Read the model definition and answer for the solid it produces. Units are mm, in the model's axes. A direction names the side the tool comes from. Give positions to 0.01 mm unless a question says otherwise; leave off trailing zeros. Loops run counter-clockwise (first coordinate to the right, second up) from the corner with the lowest first, then second, coordinate; pieces in that order, holes last.
(1) Find section A-A, the plane z = -3. Write down the section's boundary in (x, y), then the cut area to 3 significant figures.
(2) Which of the six approach directions +Z, -Z, +X, -X, +Y, -Y give full straight-line access (tool end or side, diameter ignored) to faces 5 (the face through (8.355, 10.806, -35.969)), 6 (the face through (40, 4, -56)), 7 (the face through (32.25, 2, -27)), 8 (the face through (40.2, -3.5, -31.4)), 9 (the face through (69, 3, 0))?
(3) Find section D-D, the plane z = -14. Write down the section's boundary in (x, y), then the cut area to 3 significant figures.
(4) Straight lines are drawn through the part: probe 1 along Z at (x, y) = (45.5, 4); probe 2 along X at (y, z) = (4.5, -36.5); probe 3 along Z at (x, y) = (63, 6.5). For each, find the intervals that lie inside material, in ascending order.
(5) Find section B-B, the plane x = 40. Write down the section's boundary in (y, z), then the cut area to 3 significant figures.
(6) Determine the mould class of faces 1 (the face through (78.947, 10.806, -22.671)), 2 (the face through (40, -3, -61.906)), 3 (the face through (-7.454, 3.796, -33.947)), 4 (the face through (22.52, 4.19, -42.54)) for opening direction X: pulls with the +X half, pulls with the -X half, needs draft (parallel to the pull), parting line crosses it, or undercut.
(7) Find section C-C, the plane y = -2.5. Write down the section's boundary in (x, z).
(8) Each of these flat-tipped pins is pushed along its axis until it touches: P1, Ø1.5, axis at x = 73, z = -39.5, coming from the -Y side; P2, Ø4, axis at x = 32.5, z = -20.5, coming from the +Y side; P3, Ø3, axis at y = 9.5, z = -38.5, coming from the -X side; P4, Ø3, axis at x = 11.5, y = 4.5, coming from the +Z side. Where does it stop, or does it pass through?
```python
from build123d import *

# Parameters (mm, degrees)
EXTRUDE_1_DEPTH      = 14
CUT_EXTRUDE_START    = -6.3
CUT_EXTRUDE_1_DEPTH  = 6.3
CUT_EXTRUDE_START_2  = -3
CUT_EXTRUDE_2_DEPTH  = 3
SKETCH_4_R           = 6.01
CUT_EXTRUDE_3_DEPTH  = 2.9
CUT_EXTRUDE_4_REACH  = 109.588
SKETCH_5_R           = 2.6
CUT_EXTRUDE_START_3  = -1
SKETCH_6_R           = 4.6
CUT_EXTRUDE_6_DEPTH  = 1
EXTRUDE_2_DEPTH      = 5
SKETCH_8_R           = 11.5
CUT_EXTRUDE_7_DEPTH  = 4
CUT_EXTRUDE_8_REACH  = 110.373
SKETCH_9_R           = 1.8
FILLET_1_R           = 3
SKETCH_12_R          = 10
CUT_EXTRUDE_10_DEPTH = 8
EXTRUDE_3_DEPTH      = 61.90646084
SKETCH_19_R          = 6
CUT_EXTRUDE_14_DEPTH = 9
CUT_EXTRUDE_11_REACH = 108.687
SKETCH_13_R          = 5
SKETCH_21_R          = 15
CUT_EXTRUDE_15_DEPTH = 3
SKETCH_23_R          = 1.5
CUT_EXTRUDE_16_DEPTH = 7
CUT_EXTRUDE_START_4  = -5
CUT_EXTRUDE_19_DEPTH = 5
SKETCH_34_W          = 15.5
SKETCH_34_H          = 47.251878887
CUT_EXTRUDE_20_DEPTH = 3


with BuildPart() as part:
    # 草图1 → 凸台-拉伸1 (new body)
    with BuildSketch(Plane(origin=(0, 0, 0), x_dir=(1, 0, 0), z_dir=(0, 1, 0))):
        with BuildLine():
            Line((13.709398988, 61.90646084), (-5.160444431, 39.418257154))
            ThreePointArc((-5.160444431, 39.418257154), (-7.461946981, 33.861938484), (-6.160254038, 27.990381057))
            Line((-6.160254038, 27.990381057), (10, 0))
            Line((10, 0), (70, 0))
            Line((70, 0), (86.160254038, 27.990381057))
            ThreePointArc((86.160254038, 27.990381057), (87.414448614, 34.295642979), (84.571067812, 40.061448869))
            Line((84.571067812, 40.061448869), (66.290601012, 61.90646084))
            Line((66.290601012, 61.90646084), (13.709398988, 61.90646084))
        make_face()
    extrude(amount=EXTRUDE_1_DEPTH)

    # 草图2 → 切除-拉伸1 (cut)
    with BuildSketch(Plane(origin=(0, 14, 0), x_dir=(1, 0, 0), z_dir=(0, 1, 0)).offset(CUT_EXTRUDE_START)):
        with BuildLine():
            Line((-3.314954576, 23.062177826), (1.303847577, 23.062177826))
            Line((1.303847577, 23.062177826), (12.309401077, 4))
            Line((12.309401077, 4), (67.690598923, 4))
            Line((67.690598923, 4), (78.696152423, 23.062177826))
            Line((78.696152423, 23.062177826), (83.314954576, 23.062177826))
            Line((83.314954576, 23.062177826), (86.160254038, 27.990381057))
            ThreePointArc((86.160254038, 27.990381057), (87.461946981, 33.861938484), (85.160444431, 39.418257154))
            ThreePointArc((85.160444431, 39.418257154), (84.872773368, 39.746283133), (84.571067812, 40.061448869))
            Line((84.571067812, 40.061448869), (73.343672408, 53.478096796))
            Line((73.343672408, 53.478096796), (72.5, 54.486278592))
            Line((72.5, 54.486278592), (72.5, 35.067052168))
            Line((72.5, 35.067052168), (67.5, 35.067052168))
            Line((67.5, 35.067052168), (67.5, 46.251878887))
            Line((67.5, 46.251878887), (12.5, 46.251878887))
            Line((12.5, 46.251878887), (12.5, 35.067052168))
            Line((12.5, 35.067052168), (7.5, 35.067052168))
            Line((7.5, 35.067052168), (7.5, 54.506387288))
            Line((7.5, 54.506387288), (-5.160444431, 39.418257154))
            ThreePointArc((-5.160444431, 39.418257154), (-7.461946981, 33.861938484), (-6.160254038, 27.990381057))
            Line((-6.160254038, 27.990381057), (-3.314954576, 23.062177826))
        make_face()
    extrude(amount=CUT_EXTRUDE_1_DEPTH, mode=Mode.SUBTRACT)

    # 草图3 → 切除-拉伸2 (cut)
    with BuildSketch(Plane(origin=(0, 7.7, 0), x_dir=(1, 0, 0), z_dir=(0, 1, 0)).offset(CUT_EXTRUDE_START_2)):
        with BuildLine():
            Line((67.690598923, 4), (78.696152423, 23.062177826))
            ThreePointArc((78.696152423, 23.062177826), (70.865300468, 25.508351779), (67.5, 32.990381057))
            Line((67.5, 32.990381057), (67.5, 35.067052168))
            Line((67.5, 35.067052168), (67.5, 46.251878887))
            Line((67.5, 46.251878887), (12.5, 46.251878887))
            Line((12.5, 46.251878887), (12.5, 35.067052168))
            Line((12.5, 35.067052168), (12.5, 32.990381057))
            ThreePointArc((12.5, 32.990381057), (9.134699532, 25.508351779), (1.303847577, 23.062177826))
            Line((1.303847577, 23.062177826), (12.309401077, 4))
            Line((12.309401077, 4), (67.690598923, 4))
        make_face()
    extrude(amount=CUT_EXTRUDE_2_DEPTH, mode=Mode.SUBTRACT)

    # 草图4 → 切除-拉伸3 (cut)
    with BuildSketch(Plane(origin=(0, 7.7, 0), x_dir=(1, 0, 0), z_dir=(0, 1, 0))):
        with Locations(Location((2.5, 32.990381057, 0), (0, 0, 270))):
            Circle(SKETCH_4_R)
        with Locations(Location((77.5, 32.990381057, 0), (0, 0, 270))):
            Circle(SKETCH_4_R)
    extrude(amount=-CUT_EXTRUDE_3_DEPTH, mode=Mode.SUBTRACT)

    # 草图5 → 切除-拉伸4 (cut, up to next)
    with BuildSketch(Plane(origin=(0, 4.7, 0), x_dir=(1, 0, 0), z_dir=(0, 1, 0)), mode=Mode.PRIVATE) as cut_extrude_4_sk1:
        with Locations(Location((19.414467174, 39.146743637, 0), (0, 0, 270))):
            Circle(SKETCH_5_R)
    cut_extrude_4_tool1 = extrude(cut_extrude_4_sk1.sketch, amount=-CUT_EXTRUDE_4_REACH, mode=Mode.PRIVATE) & part.part
    # 草图5 → 切除-拉伸4 (cut, up to next)
    with BuildSketch(Plane(origin=(0, 4.7, 0), x_dir=(1, 0, 0), z_dir=(0, 1, 0)), mode=Mode.PRIVATE) as cut_extrude_4_sk2:
        with Locations(Location((60.585532826, 39.146743637, 0), (0, 0, 270))):
            Circle(SKETCH_5_R)
    cut_extrude_4_tool2 = extrude(cut_extrude_4_sk2.sketch, amount=-CUT_EXTRUDE_4_REACH, mode=Mode.PRIVATE) & part.part
    add(cut_extrude_4_tool1.solids().sort_by_distance((19.414467, 4.7, -39.146744))[0], mode=Mode.SUBTRACT)
    add(cut_extrude_4_tool2.solids().sort_by_distance((60.585533, 4.7, -39.146744))[0], mode=Mode.SUBTRACT)

    # 草图6 → 切除-拉伸6 (cut)
    with BuildSketch(Plane(origin=(0, 4.7, 0), x_dir=(1, 0, 0), z_dir=(0, 1, 0)).offset(CUT_EXTRUDE_START_3)):
        with BuildLine():
            Line((67.690598923, 4), (78.696152423, 23.062177826))
            ThreePointArc((78.696152423, 23.062177826), (70.865300468, 25.508351779), (67.5, 32.990381057))
            Line((67.5, 32.990381057), (67.5, 46.251878887))
            Line((67.5, 46.251878887), (12.5, 46.251878887))
            Line((12.5, 46.251878887), (12.5, 32.990381057))
            ThreePointArc((12.5, 32.990381057), (9.134699532, 25.508351779), (1.303847577, 23.062177826))
            Line((1.303847577, 23.062177826), (12.309401077, 4))
            Line((12.309401077, 4), (67.690598923, 4))
        make_face()
        with Locations(Location((19.414467174, 39.146743637, 0), (0, 0, 270))):
            Circle(SKETCH_6_R, mode=Mode.SUBTRACT)
        with Locations(Location((60.585532826, 39.146743637, 0), (0, 0, 270))):
            Circle(SKETCH_6_R, mode=Mode.SUBTRACT)
    extrude(amount=CUT_EXTRUDE_6_DEPTH, mode=Mode.SUBTRACT)

    # 草图7 → 凸台-拉伸2 (add)
    with BuildSketch(Plane.XY):
        with BuildLine():
            Line((10, 14), (70, 14))
            ThreePointArc((70, 14), (40, -16), (10, 14))
        make_face()
    extrude(amount=EXTRUDE_2_DEPTH)

    # 草图8 → 切除-拉伸7 (cut)
    with BuildSketch(Plane.XY.offset(5)):
        with Locations((40, 14)):
            Circle(SKETCH_8_R)
    extrude(amount=-CUT_EXTRUDE_7_DEPTH, mode=Mode.SUBTRACT)

    # 草图9 → 切除-拉伸8 (cut, up to next)
    with BuildSketch(Plane(origin=(0, 0, 0), x_dir=(-1, 0, 0), z_dir=(0, 0, -1)), mode=Mode.PRIVATE) as cut_extrude_8_sk1:
        with Locations((-55, -6)):
            Circle(SKETCH_9_R)
    cut_extrude_8_tool1 = extrude(cut_extrude_8_sk1.sketch, amount=-CUT_EXTRUDE_8_REACH, mode=Mode.PRIVATE) & part.part
    # 草图9 → 切除-拉伸8 (cut, up to next)
    with BuildSketch(Plane(origin=(0, 0, 0), x_dir=(-1, 0, 0), z_dir=(0, 0, -1)), mode=Mode.PRIVATE) as cut_extrude_8_sk2:
        with Locations((-25, -6)):
            Circle(SKETCH_9_R)
    cut_extrude_8_tool2 = extrude(cut_extrude_8_sk2.sketch, amount=-CUT_EXTRUDE_8_REACH, mode=Mode.PRIVATE) & part.part
    add(cut_extrude_8_tool1.solids().sort_by_distance((55, -6, 0))[0], mode=Mode.SUBTRACT)
    add(cut_extrude_8_tool2.solids().sort_by_distance((25, -6, 0))[0], mode=Mode.SUBTRACT)

    # 圆角1
    # the kernel refuses this fillet: 3 mm, written as the material it takes off along each edge
    with BuildSketch(Plane(origin=(78.696152423, 7.7, -23.062177826), x_dir=(1, 0, 0), z_dir=(0, 1, 0))) as fillet_1_piece_1:
        with BuildLine():
            CenterArc((FILLET_1_R * 0.57735026919, -FILLET_1_R), FILLET_1_R, 90, 60)
            Line((-FILLET_1_R * 0.288675134595, -FILLET_1_R * 0.5), (0, 0))
            Line((0, 0), (FILLET_1_R * 0.57735026919, 0))
        make_face()
    extrude(amount=10.630127019, mode=Mode.SUBTRACT)
    with BuildSketch(Plane(origin=(1.303847577, 7.7, -23.062177826), x_dir=(-1, 0, 0), z_dir=(0, 1, 0))) as fillet_1_piece_2:
        with BuildLine():
            CenterArc((FILLET_1_R * 0.57735026919, FILLET_1_R), FILLET_1_R, 210, 60)
            Line((-FILLET_1_R * 0.288675134595, FILLET_1_R * 0.5), (0, 0))
            Line((0, 0), (FILLET_1_R * 0.57735026919, 0))
        make_face()
    extrude(amount=10.630127019, mode=Mode.SUBTRACT)
    with BuildSketch(Plane(origin=(7.5, 7.7, -35.067052168), x_dir=(0, 0, -1), z_dir=(0, 1, 0))) as fillet_1_piece_3:
        with BuildLine():
            CenterArc((FILLET_1_R, -FILLET_1_R), FILLET_1_R, 90, 90)
            Line((0, -FILLET_1_R), (0, 0))
            Line((0, 0), (FILLET_1_R, 0))
        make_face()
    extrude(amount=13.8, mode=Mode.SUBTRACT)
    with BuildSketch(Plane(origin=(72.5, 7.7, -35.067052168), x_dir=(0, 0, -1), z_dir=(0, 1, 0))) as fillet_1_piece_4:
        with BuildLine():
            CenterArc((FILLET_1_R, FILLET_1_R), FILLET_1_R, 180, 90)
            Line((0, FILLET_1_R), (0, 0))
            Line((0, 0), (FILLET_1_R, 0))
        make_face()
    extrude(amount=13.8, mode=Mode.SUBTRACT)

    # 草图12 → 切除-拉伸10 (cut)
    with BuildSketch(Plane(origin=(0, 0, -61.90646084), x_dir=(-1, 0, 0), z_dir=(0, 0, -1))):
        with Locations((-40, 14)):
            Circle(SKETCH_12_R)
    extrude(amount=-CUT_EXTRUDE_10_DEPTH, mode=Mode.SUBTRACT)

    # 草图16 → 凸台-拉伸3 (add)
    with BuildSketch(Plane(origin=(0, 0, -61.90646084), x_dir=(-1, 0, 0), z_dir=(0, 0, -1))):
        with BuildLine():
            ThreePointArc((-50.5, 0), (-40, -3.5), (-29.5, 0))
            Line((-29.5, 0), (-50.5, 0))
        make_face()
    extrude(amount=-EXTRUDE_3_DEPTH)

    # 草图19 → 切除-拉伸14 (cut)
    with BuildSketch(Plane.XY.offset(5)):
        with Locations((40, 14)):
            Circle(SKETCH_19_R)
    extrude(amount=-CUT_EXTRUDE_14_DEPTH, mode=Mode.SUBTRACT)

    # 草图13 → 切除-拉伸11 (cut, up to next)
    with BuildSketch(Plane(origin=(0, 0, -53.90646084), x_dir=(-1, 0, 0), z_dir=(0, 0, -1)), mode=Mode.PRIVATE) as cut_extrude_11_sk1:
        with Locations((-40, 14)):
            Circle(SKETCH_13_R)
    cut_extrude_11_tool1 = extrude(cut_extrude_11_sk1.sketch, amount=-CUT_EXTRUDE_11_REACH, mode=Mode.PRIVATE) & part.part
    add(cut_extrude_11_tool1.solids().sort_by_distance((40, 14, -53.906461))[0], mode=Mode.SUBTRACT)

    # 草图21 → 切除-拉伸15 (cut)
    with BuildSketch(Plane(origin=(0, 0, -61.90646084), x_dir=(-1, 0, 0), z_dir=(0, 0, -1))):
        with Locations((-40, 14)):
            Circle(SKETCH_21_R)
    extrude(amount=-CUT_EXTRUDE_15_DEPTH, mode=Mode.SUBTRACT)

    # 草图23 → 切除-拉伸16 (cut)
    with BuildSketch(Plane(origin=(0, 0, -58.90646084), x_dir=(-1, 0, 0), z_dir=(0, 0, -1))):
        with Locations((-50.356157589, 7)):
            Circle(SKETCH_23_R)
        with Locations((-29.643842411, 7)):
            Circle(SKETCH_23_R)
    extrude(amount=-CUT_EXTRUDE_16_DEPTH, mode=Mode.SUBTRACT)

    # 草图33 → 切除-拉伸19 (cut)
    with BuildSketch(Plane.XY.offset(-46.251878887).offset(CUT_EXTRUDE_START_4)):
        with BuildLine():
            Line((35, 14), (12.5, 14))
            Line((12.5, 14), (12.5, 3.7))
            Line((12.5, 3.7), (67.5, 3.7))
            Line((67.5, 3.7), (67.5, 14))
            Line((67.5, 14), (45, 14))
            ThreePointArc((45, 14), (40, 9), (35, 14))
        make_face()
    extrude(amount=CUT_EXTRUDE_19_DEPTH, mode=Mode.SUBTRACT)

    # 草图34 → 切除-拉伸20 (cut)
    with BuildSketch(Plane(origin=(0, 3.7, 0), x_dir=(1, 0, 0), z_dir=(0, 1, 0))):
        with Locations((40, 27.625939444)):
            Rectangle(SKETCH_34_W, SKETCH_34_H)
    extrude(amount=-CUT_EXTRUDE_20_DEPTH, mode=Mode.SUBTRACT)


solid = part.part
```
Entries:
1. outline: (8.27, 0) - (29.5, 0) arc R17.5 ccw to (50.5, 0) - (71.73, 0) - (71.73, 14) - (46, 14) arc R6 cw to (34, 14) - (8.27, 14) - close
1. area: 882 mm2
2. face 5: -X, +Y
2. face 6: -Z, +Y
2. face 7: +Y
2. face 8: -Z, -Y
2. face 9: +Z, +X, -Y
3. outline: (1.92, 0) - (29.5, 0) arc R17.5 ccw to (50.5, 0) - (78.08, 0) - (78.08, 14) - (73.46, 14) - (73.46, 3.7) - (47.75, 3.7) - (47.75, 0.7) - (32.25, 0.7) - (32.25, 3.7) - (6.54, 3.7) - (6.54, 14) - (1.92, 14) - close
3. area: 381 mm2
4. probe 1: z = -58.91 to -51.25, -4 to 1
4. probe 2: x = -6.86 to 12.5, 15.65 to 23.18, 56.82 to 64.35, 67.5 to 86.86
4. probe 3: z = -61.91 to -51.25, -4 to 5
5. outline: (-16, 0) - (-3.5, 0) - (-3.5, -61.91) - (-1, -61.91) - (-1, -58.91) - (4, -58.91) - (4, -53.91) - (9, -53.91) - (9, -51.25) - (0.7, -51.25) - (0.7, -4) - (8, -4) - (8, 1) - (2.5, 1) - (2.5, 5) - (-16, 5) - close
5. area: 421 mm2
6. face 1: undercut
6. face 2: needs draft
6. face 3: pulls with the -X half
6. face 4: undercut
7. outline: (14.95, 0) - (34.17, 0) - (34.17, -61.91) - (45.83, -61.91) - (45.83, 0) - (65.05, 0) - (65.05, 5) - (14.95, 5) - close
8. P1: stops at y = 0
8. P2: stops at y = 3.7
8. P3: stops at x = 7.5
8. P4: stops at z = 5
